Read the model definition and answer for the solid it produces. Units are mm, in the model's axes. A direction names the side the tool comes from. Coordinates: 2 decimals unless noted, no trailing zeros. Loops run counter-clockwise (first coordinate to the right, second up) from the corner with the lowest first, then second, coordinate; pieces in that order, holes last.
from build123d import *

# Parameters (mm, degrees)
BOX036_W     = 6
BOX036_H     = 4
BOX036_DEPTH = 1
BOX027_W     = 45
BOX027_H     = 25
BOX027_DEPTH = 1


with BuildPart() as box036:
    # Box036 → Box036 (new body)
    with BuildSketch(Plane(origin=(1, 1, 10), x_dir=(1, 0, 0), z_dir=(0, 0, 1))):
        with Locations((3, 2)):
            Rectangle(BOX036_W, BOX036_H)
    extrude(amount=BOX036_DEPTH)


with BuildPart() as cut038:
    # Box027 → Box027 (new body)
    with BuildSketch(Plane.XY.offset(10)):
        with Locations((22.5, 12.5)):
            Rectangle(BOX027_W, BOX027_H)
    extrude(amount=BOX027_DEPTH)

    # Cut038: cut Box036
    add(box036.part, mode=Mode.SUBTRACT)


solid = cut038.part
Item 1: A cutting plane is placed at B-B on z = 10.85. Determine the outline of the cut face in (x, y).
Numbers:
outline: (0, 0) - (45, 0) - (45, 25) - (0, 25) - close; hole (1, 1) - (7, 1) - (7, 5) - (1, 5) - close
Item 2: Determine the mould class of faces 3 (the face through (4, 5, 10.5)), 4 (the face through (1, 3, 10.5)), 5 (the face through (22.2, 0, 10.5)), 6 (the face through (0, 12.3, 10.5)) for opening direction X: released by +X, released by -X, zero draft, split by the parting line, or undercut.
Numbers:
face 3: undercut
face 4: undercut
face 5: zero draft
face 6: released by -X
Item 3: Find the intervals of material crossed by line 1 along Y through (x, z) = (4, 10.45); line 2 along X through (y, z) = (2.25, 10.5), in increasing order.
Numbers:
line 1: y = 0 to 1, 5 to 25
line 2: x = 0 to 1, 7 to 45
Item 4: Which of the six approach directions +Z, -Z, +X, -X, +Y, -Y give full straight-line access (tool end or side, diameter ignored) to faces 1 (the face through (22, 13, 10)), 2 (the face through (7, 3, 10.5))?
Numbers:
face 1: -Z, +X, -X, +Y, -Y
face 2: +Z, -Z
Item 5: A cutting plane is placed at A-A on y = 4.5. Determine the outline of the cut face in (x, z), then the cut area to 3 significant figures.
Numbers:
outline: (0, 10) - (1, 10) - (1, 11) - (0, 11) - close; (7, 10) - (45, 10) - (45, 11) - (7, 11) - close
area: 39.0 mm2
